```python
from build123d import *

# Parameters (mm, degrees)
SKETCH1_W                       = 56
SKETCH1_H                       = 40
BOSS_EXTRUDE1_DEPTH             = 10
SKETCH2_W                       = 13
SKETCH2_H                       = 32.863436123
CUT_EXTRUDE1_DEPTH              = 55.723267722
SKETCH3_W                       = 13
SKETCH3_H                       = 32.863436123
CUT_EXTRUDE2_DEPTH              = 55.723267722
F_14_0_14_DIAMETER_HOLE1_D      = 14
F_3_3_3_3_DIAMETER_HOLE1_REACH  = 58.473
F_3_3_3_3_DIAMETER_HOLE1_BORE_R = 1.65
F_5_0_5_DIAMETER_HOLE1_D        = 5
CHAMFER1_SIZE                   = 2
FILLET1_R                       = 1


with BuildPart() as part:
    # Sketch1 → Boss-Extrude1 (new body)
    with BuildSketch(Plane.XY.offset(10)):
        with Locations((-10.59030837, 17.488986784)):
            Rectangle(SKETCH1_W, SKETCH1_H)
    extrude(amount=-BOSS_EXTRUDE1_DEPTH)

    # Sketch2 → Cut-Extrude1 (cut, through all)
    with BuildSketch(Plane(origin=(0, 0, 0), x_dir=(-1, 0, 0), z_dir=(0, 0, -1))):
        with Locations((32.09030837, 21.057268723)):
            Rectangle(SKETCH2_W, SKETCH2_H)
    extrude(amount=-CUT_EXTRUDE1_DEPTH, mode=Mode.SUBTRACT)

    # Sketch3 → Cut-Extrude2 (cut, through all)
    with BuildSketch(Plane(origin=(0, 0, 0), x_dir=(-1, 0, 0), z_dir=(0, 0, -1))):
        with Locations((-10.90969163, 21.057268723)):
            Rectangle(SKETCH3_W, SKETCH3_H)
    extrude(amount=-CUT_EXTRUDE2_DEPTH, mode=Mode.SUBTRACT)

    # Ø14.0 (14) Diameter Hole1 (through all)
    with Locations(Plane.XY.offset(10)):
        with Locations((-10.59030837, 22.488986784)):
            Hole(F_14_0_14_DIAMETER_HOLE1_D / 2)

    # Ø3.3 (3.3) Diameter Hole1 bore → Ø3.3 (3.3) Diameter Hole1 (cut, up to next)
    with BuildSketch(Plane(origin=(0, 37.488986784, 0), x_dir=(1, 0, 0), z_dir=(0, 1, 0)), mode=Mode.PRIVATE) as f_3_3_3_3_diameter_hole1_sk1:
        with Locations((-10.59030837, -5)):
            Circle(F_3_3_3_3_DIAMETER_HOLE1_BORE_R)
    f_3_3_3_3_diameter_hole1_tool1 = extrude(f_3_3_3_3_diameter_hole1_sk1.sketch, amount=-F_3_3_3_3_DIAMETER_HOLE1_REACH, mode=Mode.PRIVATE) & part.part
    add(f_3_3_3_3_diameter_hole1_tool1.solids().sort_by_distance((-10.590308, 37.488987, 5))[0], mode=Mode.SUBTRACT)

    # Ø5.0 (5) Diameter Hole1 (through all)
    with Locations(Plane(origin=(0, 4.625550661, 0), x_dir=(1, 0, 0), z_dir=(0, 1, 0))):
        with Locations((-32.09030837, -5), (10.90969163, -5)):
            Hole(F_5_0_5_DIAMETER_HOLE1_D / 2)

    # Chamfer1
    chamfer1_edges = [part.edges().sort_by_distance(p)[0] for p in [
        (-25.59030837, 37.488986784, 5),
        (4.40969163, 37.488986784, 5),
    ]]
    chamfer(chamfer1_edges, length=CHAMFER1_SIZE)

    # Fillet1
    fillet1_edges = [part.edges().sort_by_distance(p)[0] for p in [
        (17.40969163, 1.057268722, 0),
        (-38.59030837, 1.057268722, 10),
        (-38.59030837, 1.057268722, 0),
        (17.40969163, 1.057268722, 10),
    ]]
    fillet(fillet1_edges, radius=FILLET1_R)


solid = part.part
```
Work out the finished part from the listing and answer in its coordinate system (mm). A direction names the side the tool comes from. Coordinates: 2 decimals unless noted, no trailing zeros. Loops run counter-clockwise (first coordinate to the right, second up) from the corner with the lowest first, then second, coordinate; pieces in that order, holes last. Notation, with made-up numbers: M 85,73.5 L 112,73.5 A20 ccw 112,84.5 Z; hole C 30,60 d6. An arc over 180 degrees is marked long. Use CSV: the item, a comma, the result in double quotes. Start each with the question number.
(1) For a pull along Y with two mould halves and no side action, classify faces 1 (the face through (-11, 37.489, 7)), 2 (the face through (4.41, 20, 5)), 3 (the face through (-13.82, 16.28, 4.93)) as +Y half, -Y half, draft (parallel to the pull), parting line (faces both ways), or undercut.
(2) Find section D-D, the plane y = 8.5. Give the vertices of the cut face in (x, z).
(3) For faces 4 (the face through (-25.59, 20, 5)), 5 (the face through (9.56, 4.626, 2.71)), 6 (the face through (-9.066, 33.445, 5.632)), 7 (the face through (-11, -2.511, 5)), 8 (the face through (17.41, 1, 5)), determine the directions among +Z, -Z, +X, -X, +Y, -Y from which every point of the face is accessible in a straight line to the end or side of a thin tool.
(4) Consider line 1 (X direction, y = 4.5, z = 7); line 2 (X direction, y = 32, z = 5); line 3 (X direction, y = 1, z = 4.25). Determine where each line is inside the solid, lowest interval first.
(5) Find section B-B, the plane x = -31.5. Give the vertices of the cut face in (y, z).
(6) Find section C-C, the plane y = 26. Give the vertices of the cut face in (x, z).
(7) Find section A-A, the plane z = 5. Give the vertices of the cut face in (x, y), then the cut area to 3 significant figures.
(8) Given pin 1 Ø1.5 at (y, z) = (8, 4) entering from +X; pin 2 Ø3 at (y, z) = (18, 1.5) entering from -X; pin 3 Ø3 at (x, z) = (9, 5.5) entering from +Y; pin 4 Ø4 at (x, z) = (-32.09, 5) entering from -Y, each flat-ended and moving along its own axis, determine where each tip first touches the part or whether it passes through.
Recorded:
1,face 1,"+Y half"
1,face 2,"draft"
1,face 3,"undercut"
2,outline,"M -25.59,0 L 4.41,0 L 4.41,10 L -25.59,10 Z"
3,face 4,"+Z, -Z, -X, +Y"
3,face 5,"+Z, -Z, +X, +Y"
3,face 6,"+Y"
3,face 7,"+Z, -Z, +X, -X, -Y"
3,face 8,"+Z, -Z, +X, +Y, -Y"
4,line 1,"x = -38.59 to -33.59, -30.59 to 9.41, 12.41 to 17.41"
4,line 2,"x = -25.59 to -12.24, -8.94 to 4.41"
4,line 3,"x = -38.59 to -34.48, -29.71 to 8.52, 13.29 to 17.41"
5,outline,"M -2.51,0 L 4.63,0 L 4.63,2.57 L -2.51,2.57 Z; M -2.51,7.43 L 4.63,7.43 L 4.63,10 L -2.51,10 Z"
6,outline,"M -25.59,0 L -16.65,0 L -16.65,10 L -25.59,10 Z; M -4.53,0 L 4.41,0 L 4.41,10 L -4.53,10 Z"
7,outline,"M -38.59,-2.51 L -34.59,-2.51 L -34.59,4.63 L -38.59,4.63 Z; M -29.59,-2.51 L 8.41,-2.51 L 8.41,4.63 L 4.41,4.63 L 4.41,35.49 L 2.41,37.49 L -8.94,37.49 L -8.94,29.29 A7 cw long -12.24,29.29 L -12.24,37.49 L -23.59,37.49 L -25.59,35.49 L -25.59,4.63 L -29.59,4.63 Z; M 13.41,-2.51 L 17.41,-2.51 L 17.41,4.63 L 13.41,4.63 Z"
7,area,"1,130 mm^2"
8,pin 1,"stops at x = 4.41"
8,pin 2,"stops at x = -25.59"
8,pin 3,"stops at y = 4.63"
8,pin 4,"passes through"
